```python
from build123d import *

# Parameters (mm, degrees)
SKETCH1_W           = 420
SKETCH1_H           = 110
BOSS_EXTRUDE1_DEPTH = 2
CUT_EXTRUDE1_REACH  = 4
SKETCH2_R           = 3
CUT_EXTRUDE2_REACH  = 4
SKETCH3_R           = 3
SKETCH3_R_2         = 2.5
SKETCH3_W           = 47.5
SKETCH3_H           = 28
FILLET1_R           = 2


with BuildPart() as part:
    # Sketch1 → Boss-Extrude1 (new body)
    with BuildSketch(Plane.ZY.offset(26.051745534)):
        with Locations((184.692172039, 45)):
            Rectangle(SKETCH1_W, SKETCH1_H)
    extrude(amount=BOSS_EXTRUDE1_DEPTH)

    # Sketch2 → Cut-Extrude1 (cut, up to next)
    with BuildSketch(Plane.ZY.offset(28.051745534), mode=Mode.PRIVATE) as cut_extrude1_sk1:
        with Locations((-20.307827961, 75)):
            Circle(SKETCH2_R)
    cut_extrude1_tool1 = extrude(cut_extrude1_sk1.sketch, amount=-CUT_EXTRUDE1_REACH, mode=Mode.PRIVATE) & part.part
    add(cut_extrude1_tool1.solids().sort_by_distance((-28.051746, 75, -20.307828))[0], mode=Mode.SUBTRACT)
    # Sketch2 → Cut-Extrude1 (cut, up to next)
    with BuildSketch(Plane.ZY.offset(28.051745534), mode=Mode.PRIVATE) as cut_extrude1_sk2:
        with Locations((-20.307827961, 25)):
            Circle(SKETCH2_R)
    cut_extrude1_tool2 = extrude(cut_extrude1_sk2.sketch, amount=-CUT_EXTRUDE1_REACH, mode=Mode.PRIVATE) & part.part
    add(cut_extrude1_tool2.solids().sort_by_distance((-28.051746, 25, -20.307828))[0], mode=Mode.SUBTRACT)
    # Sketch2 → Cut-Extrude1 (cut, up to next)
    with BuildSketch(Plane.ZY.offset(28.051745534), mode=Mode.PRIVATE) as cut_extrude1_sk3:
        with Locations((389.692172039, 75)):
            Circle(SKETCH2_R)
    cut_extrude1_tool3 = extrude(cut_extrude1_sk3.sketch, amount=-CUT_EXTRUDE1_REACH, mode=Mode.PRIVATE) & part.part
    add(cut_extrude1_tool3.solids().sort_by_distance((-28.051746, 75, 389.692172))[0], mode=Mode.SUBTRACT)
    # Sketch2 → Cut-Extrude1 (cut, up to next)
    with BuildSketch(Plane.ZY.offset(28.051745534), mode=Mode.PRIVATE) as cut_extrude1_sk4:
        with Locations((389.692172039, 25)):
            Circle(SKETCH2_R)
    cut_extrude1_tool4 = extrude(cut_extrude1_sk4.sketch, amount=-CUT_EXTRUDE1_REACH, mode=Mode.PRIVATE) & part.part
    add(cut_extrude1_tool4.solids().sort_by_distance((-28.051746, 25, 389.692172))[0], mode=Mode.SUBTRACT)

    # Sketch3 → Cut-Extrude2 (cut, up to next)
    with BuildSketch(Plane.ZY.offset(28.051745534), mode=Mode.PRIVATE) as cut_extrude2_sk1:
        with Locations((94.692172039, 10)):
            Circle(SKETCH3_R)
    cut_extrude2_tool1 = extrude(cut_extrude2_sk1.sketch, amount=-CUT_EXTRUDE2_REACH, mode=Mode.PRIVATE) & part.part
    add(cut_extrude2_tool1.solids().sort_by_distance((-28.051746, 10, 94.692172))[0], mode=Mode.SUBTRACT)
    # Sketch3 → Cut-Extrude2 (cut, up to next)
    with BuildSketch(Plane.ZY.offset(28.051745534), mode=Mode.PRIVATE) as cut_extrude2_sk2:
        with Locations((274.692172039, 10)):
            Circle(SKETCH3_R)
    cut_extrude2_tool2 = extrude(cut_extrude2_sk2.sketch, amount=-CUT_EXTRUDE2_REACH, mode=Mode.PRIVATE) & part.part
    add(cut_extrude2_tool2.solids().sort_by_distance((-28.051746, 10, 274.692172))[0], mode=Mode.SUBTRACT)
    # Sketch3 → Cut-Extrude2 (cut, up to next)
    with BuildSketch(Plane.ZY.offset(28.051745534), mode=Mode.PRIVATE) as cut_extrude2_sk3:
        with Locations((94.692172039, 80)):
            Circle(SKETCH3_R)
    cut_extrude2_tool3 = extrude(cut_extrude2_sk3.sketch, amount=-CUT_EXTRUDE2_REACH, mode=Mode.PRIVATE) & part.part
    add(cut_extrude2_tool3.solids().sort_by_distance((-28.051746, 80, 94.692172))[0], mode=Mode.SUBTRACT)
    # Sketch3 → Cut-Extrude2 (cut, up to next)
    with BuildSketch(Plane.ZY.offset(28.051745534), mode=Mode.PRIVATE) as cut_extrude2_sk4:
        with Locations((274.692172039, 80)):
            Circle(SKETCH3_R)
    cut_extrude2_tool4 = extrude(cut_extrude2_sk4.sketch, amount=-CUT_EXTRUDE2_REACH, mode=Mode.PRIVATE) & part.part
    add(cut_extrude2_tool4.solids().sort_by_distance((-28.051746, 80, 274.692172))[0], mode=Mode.SUBTRACT)
    # Sketch3 → Cut-Extrude2 (cut, up to next)
    with BuildSketch(Plane.ZY.offset(28.051745534), mode=Mode.PRIVATE) as cut_extrude2_sk5:
        with Locations((359.1226293, 94)):
            Circle(SKETCH3_R_2)
    cut_extrude2_tool5 = extrude(cut_extrude2_sk5.sketch, amount=-CUT_EXTRUDE2_REACH, mode=Mode.PRIVATE) & part.part
    add(cut_extrude2_tool5.solids().sort_by_distance((-28.051746, 94, 359.122629))[0], mode=Mode.SUBTRACT)
    # Sketch3 → Cut-Extrude2 (cut, up to next)
    with BuildSketch(Plane.ZY.offset(28.051745534), mode=Mode.PRIVATE) as cut_extrude2_sk6:
        with Locations((308.3226293, 79)):
            Circle(SKETCH3_R_2)
    cut_extrude2_tool6 = extrude(cut_extrude2_sk6.sketch, amount=-CUT_EXTRUDE2_REACH, mode=Mode.PRIVATE) & part.part
    add(cut_extrude2_tool6.solids().sort_by_distance((-28.051746, 79, 308.322629))[0], mode=Mode.SUBTRACT)
    # Sketch3 → Cut-Extrude2 (cut, up to next)
    with BuildSketch(Plane.ZY.offset(28.051745534), mode=Mode.PRIVATE) as cut_extrude2_sk7:
        with Locations((308.3226293, 50.4)):
            Circle(SKETCH3_R_2)
    cut_extrude2_tool7 = extrude(cut_extrude2_sk7.sketch, amount=-CUT_EXTRUDE2_REACH, mode=Mode.PRIVATE) & part.part
    add(cut_extrude2_tool7.solids().sort_by_distance((-28.051746, 50.4, 308.322629))[0], mode=Mode.SUBTRACT)
    # Sketch3 → Cut-Extrude2 (cut, up to next)
    with BuildSketch(Plane.ZY.offset(28.051745534), mode=Mode.PRIVATE) as cut_extrude2_sk8:
        with Locations((359.1226293, 46.4)):
            Circle(SKETCH3_R_2)
    cut_extrude2_tool8 = extrude(cut_extrude2_sk8.sketch, amount=-CUT_EXTRUDE2_REACH, mode=Mode.PRIVATE) & part.part
    add(cut_extrude2_tool8.solids().sort_by_distance((-28.051746, 46.4, 359.122629))[0], mode=Mode.SUBTRACT)
    # Sketch3 → Cut-Extrude2 (cut, up to next)
    with BuildSketch(Plane.ZY.offset(28.051745534), mode=Mode.PRIVATE) as cut_extrude2_sk9:
        with Locations((48.442172039, 19)):
            Rectangle(SKETCH3_W, SKETCH3_H)
    cut_extrude2_tool9 = extrude(cut_extrude2_sk9.sketch, amount=-CUT_EXTRUDE2_REACH, mode=Mode.PRIVATE) & part.part
    add(cut_extrude2_tool9.solids().sort_by_distance((-28.051746, 19, 48.442172))[0], mode=Mode.SUBTRACT)

    # Fillet1
    fillet1_edges = [part.edges().sort_by_distance(p)[0] for p in [
        (-27.051745534, 5, 24.692172039),
        (-27.051745534, 33, 24.692172039),
        (-27.051745534, 33, 72.192172039),
        (-27.051745534, 5, 72.192172039),
    ]]
    fillet(fillet1_edges, radius=FILLET1_R)


solid = part.part
```
Part model, mm, in its own coordinate system. Round coordinates to 2 decimals unless told otherwise and drop trailing zeros. Order: outer loops, then holes, each group sorted by start corner. A loop starts at its lowest first (then second) coordinate and runs counter-clockwise, first axis right, second up. Notation, with made-up numbers: M 72.5,76 L 114.5,76 A18 ccw 114.5,107 Z; hole C 79,20 d2. An arc over 180 degrees is marked long. Answer in a Markdown table with one row per item. Add a question column.
Q1. Cut at A-A on z = 34.5. Give the cut face in (x, y), and give its area (3 significant figures).
Q2. Cut at B-B on x = -27.35. Give the number of separate pieces and of enclosed holes in the cut face, and give its area (3 significant figures).
Q3. Wall check: L1, parallel to Z at x = -26.8, y = 31.5; L2, parallel to Z at x = -27.3, y = 30; L3, parallel to Y at x = -26.6, z = 68.5. Give the ranges that are in metal, low to high. Write a range as from..to.
Q4. Pin check, flat tip, straight feed: pin 1 (3.5 mm diameter, centred on y = 75, z = 389.69, fed in from -X). Stop position of the tip, or through.
Established:
| question | item | result |
|---|---|---|
| 1 | outline | M -28.05,-10 L -26.05,-10 L -26.05,5 L -28.05,5 Z; M -28.05,33 L -26.05,33 L -26.05,100 L -28.05,100 Z |
| 1 | area | 164 mm2 |
| 2 | separate pieces | 1 |
| 2 | enclosed holes | 13 |
| 2 | area | 44,600 mm2 |
| 3 | L1 | z = -25.31..24.76, 72.13..394.69 |
| 3 | L2 | z = -25.31..24.69, 72.19..394.69 |
| 3 | L3 | y = -10..5, 33..100 |
| 4 | pin 1 | passes through |
